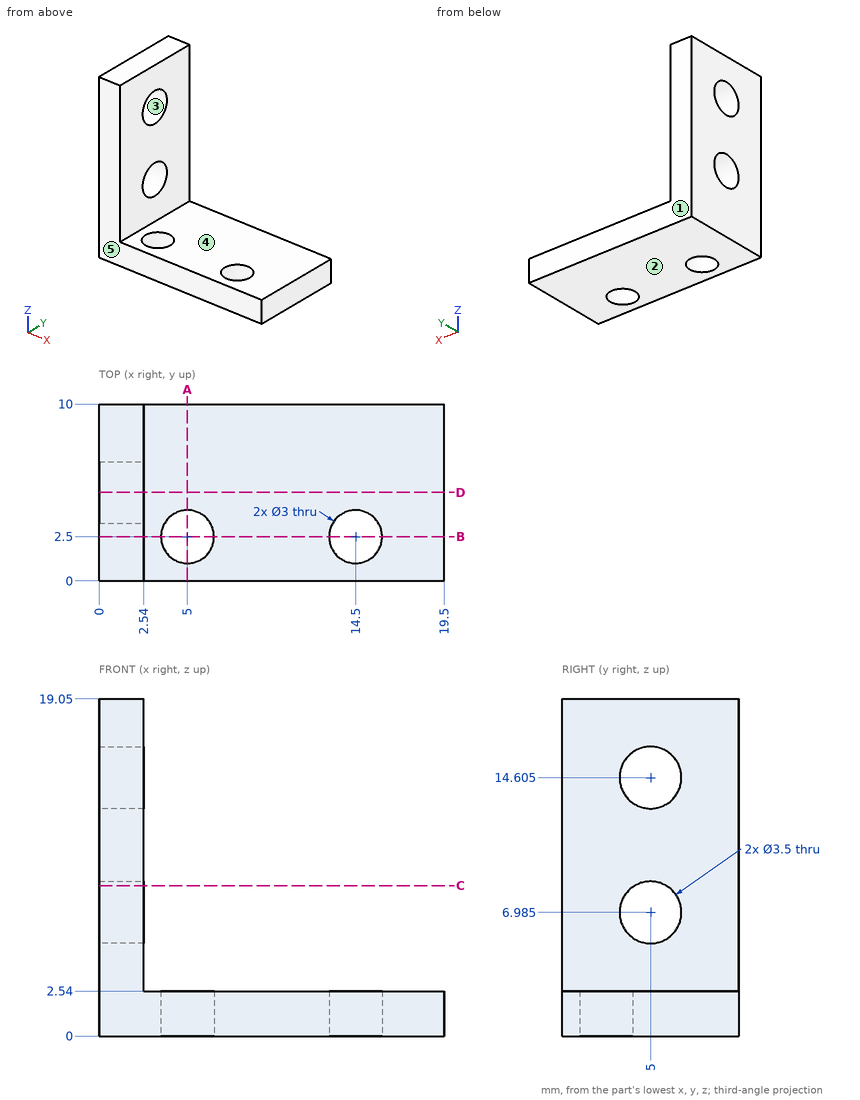
Can you work these out from the drawing? Everything is in mm from the part's minimum corner. A direction names the side the tool comes from. Round coordinates to 2 decimals unless told otherwise and drop trailing zeros. Loops run counter-clockwise (first coordinate to the right, second up) from the corner with the lowest first, then second, coordinate; pieces in that order, holes last. Notation, with made-up numbers: M 60.25,25 L 106.25,25 A17 ccw 106.25,48 Z; hole C 60,-16.75 d2. An arc over 180 degrees is marked long. Answer in a Markdown table with one row per item.
1. Thinking about a two-plate mould opening in Z: for the marked faces 1, 2 and 3, which applies, pulls with the +Z half, pulls with the -Z half, needs draft (parallel to the pull), parting line crosses it, or undercut?
Established:
| item | result |
|---|---|
| face 1 | needs draft |
| face 2 | pulls with the -Z half |
| face 3 | undercut |
2. If we section it at D-D, the plane y = 5: Please give me the cut outline in (x, z) (3 decimals), plus the area to 3 significant figures.
Established:
| item | result |
|---|---|
| outline | M 0,0 L 19.5,0 L 19.5,2.54 L 2.54,2.54 L 2.54,5.235 L 0,5.235 Z; M 0,8.735 L 2.54,8.735 L 2.54,12.855 L 0,12.855 Z; M 0,16.355 L 2.54,16.355 L 2.54,19.05 L 0,19.05 Z |
| area | 73.7 mm² |
3. I'm going to push flat-ended pins straight in: pin 1 Ø5 at (y, z) = (4.5, 13.5) entering from +X; pin 2 Ø4 at (y, z) = (7, 12) entering from -X; pin 3 Ø5 at (x, y) = (14.5, 2.5) entering from +Z. Where does each tip first touch, or does it pass through?
Established:
| item | result |
|---|---|
| pin 1 | x = 2.54 |
| pin 2 | x = 0 |
| pin 3 | z = 2.54 |
4. If we section it at C-C, the plane z = 8.5: Please give me the cut outline in (x, y), plus the area to 3 significant figures.
Established:
| item | result |
|---|---|
| outline | M 0,0 L 2.54,0 L 2.54,4.12 L 0,4.12 Z; M 0,5.88 L 2.54,5.88 L 2.54,10 L 0,10 Z |
| area | 21.0 mm² |
5. Please list where these lines run through material, in increasing order: line 1 (X direction, y = 9.5, z = 8.5); line 2 (Y direction, x = 5, z = 1). Write a range as from..to.
Established:
| item | result |
|---|---|
| line 1 | 0..2.54 |
| line 2 | 0..1, 4..10 |
6. If we section it at A-A, the plane x = 5: Please give me the cut outline in (y, z), plus the area to 3 significant figures.
Established:
| item | result |
|---|---|
| outline | M 0,0 L 1,0 L 1,2.54 L 0,2.54 Z; M 4,0 L 10,0 L 10,2.54 L 4,2.54 Z |
| area | 17.8 mm² |
7. If we section it at B-B, the plane y = 2.5: Please give me the cut outline in (x, z), plus the area to 3 significant figures.
Established:
| item | result |
|---|---|
| outline | M 0,0 L 3.5,0 L 3.5,2.54 L 2.54,2.54 L 2.54,19.05 L 0,19.05 Z; M 6.5,0 L 13,0 L 13,2.54 L 6.5,2.54 Z; M 16,0 L 19.5,0 L 19.5,2.54 L 16,2.54 Z |
| area | 76.2 mm² |
8. On a 3-axis mill with a long thin cutter (end or side, diameter ignored), from which of +Z, -Z, +X, -X, +Y, -Y can I reach the whole of each face in a straight line? I mean the marked faces 4 and 5. Say none if no direction works.
Established:
| item | result |
|---|---|
| face 4 | +Z, +X, +Y, -Y |
| face 5 | +Z, -Z, +X, -X, -Y |
